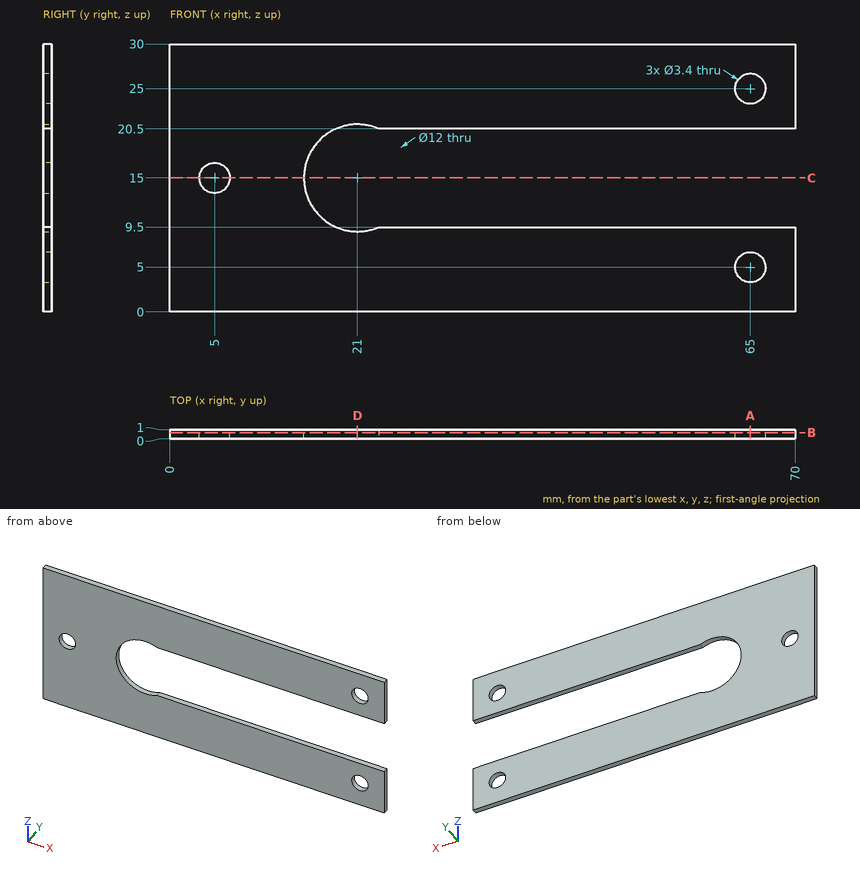
Source: three-view drawing plus pictorial views. Frame: mm from the lowest corner of the part. Round coordinates to 2 decimals unless told otherwise and drop trailing zeros. Loops run counter-clockwise (first coordinate to the right, second up) from the corner with the lowest first, then second, coordinate; pieces in that order, holes last. Notation, with made-up numbers: M 80,61 L 110,61 A30 ccw 110,89 Z; hole C 46.5,-23 d4. An arc over 180 degrees is marked long. Put each result on its own line as item: value. Start each with the question number.
(1) Section query C-C (z = 15). Return loops of the section in (x, y).
(2) Material intervals for line 1 along Z through (x, y) = (33.5, 0.15); line 2 along X through (y, z) = (0.55, 25); line 3 along Z through (x, y) = (21, 0.3), sorted ascending. Write a range as [from, to].
(3) Section query D-D (x = 21). Return loops of the section in (y, z), then the cut area to 3 significant figures.
(4) Section query B-B (y = 0.7). Return loops of the section in (x, z).
(5) Section query A-A (x = 65). Return loops of the section in (y, z), then the cut area to 3 significant figures.
(6) Contact query for a flat-ended pin moving along its axis: pin 1 Ø3 at (x, z) = (65, 25) entering from +Y. Output: stop coordinate, or through.
Findings below:
1. outline: M 0,0 L 3.3,0 L 3.3,1 L 0,1 Z; M 6.7,0 L 15,0 L 15,1 L 6.7,1 Z
2. line 1: z = [0, 9.5], [20.5, 30]
2. line 2: x = [0, 63.3], [66.7, 70]
2. line 3: z = [0, 9], [21, 30]
3. outline: M 0,0 L 1,0 L 1,9 L 0,9 Z; M 0,21 L 1,21 L 1,30 L 0,30 Z
3. area: 18.0 mm2
4. outline: M 0,0 L 70,0 L 70,9.5 L 23.4,9.5 A6 cw long 23.4,20.5 L 70,20.5 L 70,30 L 0,30 Z; hole C 5,15 d3.4; hole C 65,5 d3.4; hole C 65,25 d3.4
5. outline: M 0,0 L 1,0 L 1,3.3 L 0,3.3 Z; M 0,6.7 L 1,6.7 L 1,9.5 L 0,9.5 Z; M 0,20.5 L 1,20.5 L 1,23.3 L 0,23.3 Z; M 0,26.7 L 1,26.7 L 1,30 L 0,30 Z
5. area: 12.2 mm2
6. pin 1: passes through
